```python
from build123d import *

# Parameters (mm, degrees)
EXTRUDE_1_DEPTH      = 3
EXTRUDE_1_DEPTH_BACK = 3
SKETCH_2_W           = 0.5
SKETCH_2_H           = 3
SKETCH_2_H_2         = 1.25
EXTRUDE_2_DEPTH      = 35
SKETCH_3_W           = 6
SKETCH_3_H           = 3
CUT_EXTRUDE_1_DEPTH  = 1.5
CUT_EXTRUDE_2_REACH  = 31.123
SKETCH_4_W           = 0.75
SKETCH_4_H           = 3
SKETCH_2_4_W         = 0.5
SKETCH_2_4_H         = 1.25
EXTRUDE_3_DEPTH      = 4
EXTRUDE_4_REACH      = 40.773
SKETCH_5_W           = 3
SKETCH_5_H           = 3


with BuildPart() as part:
    # Sketch 1 → Extrude 1 (new, two sides: drawn at the far end of the back side and taken through both)
    with BuildSketch(Plane(origin=(0, 0, 0), x_dir=(1, 0, 0), z_dir=(0, 1, 0)).offset(-EXTRUDE_1_DEPTH_BACK)):
        Polygon((-14.75, -19.75), (-14.75, 19.75), (14.75, 19.75), (14.75, -19.75), (15.75, -19.75), (15.75, 23.75), (-15.75, 23.75), (-15.75, -19.75), align=None)
    extrude(amount=EXTRUDE_1_DEPTH + EXTRUDE_1_DEPTH_BACK)

    # Sketch 2 → Extrude 2 (add)
    with BuildSketch(Plane.XY.offset(-19.75)):
        with Locations((-14.5, -1.5)):
            Rectangle(SKETCH_2_W, SKETCH_2_H)
        with Locations((-14.5, 2.375)):
            Rectangle(SKETCH_2_W, SKETCH_2_H_2)
        with Locations((14.5, -1.5)):
            Rectangle(SKETCH_2_W, SKETCH_2_H)
    extrude(amount=EXTRUDE_2_DEPTH)

    # Sketch 3 → Cut-Extrude 1 (cut)
    with BuildSketch(Plane(origin=(0, 0, -23.75), x_dir=(-1, 0, 0), z_dir=(0, 0, -1))):
        with Locations((-9.25, -1.5)):
            Rectangle(SKETCH_3_W, SKETCH_3_H)
        with Locations((9.25, -1.5)):
            Rectangle(SKETCH_3_W, SKETCH_3_H)
    extrude(amount=-CUT_EXTRUDE_1_DEPTH, mode=Mode.SUBTRACT)

    # Sketch 4 → Cut-Extrude 2 (cut, up to next)
    with BuildSketch(Plane(origin=(0, 3, 0), x_dir=(1, 0, 0), z_dir=(0, 1, 0)), mode=Mode.PRIVATE) as cut_extrude_2_sk1:
        with Locations((-15.375, 22.25)):
            Rectangle(SKETCH_4_W, SKETCH_4_H)
    cut_extrude_2_tool1 = extrude(cut_extrude_2_sk1.sketch, amount=-CUT_EXTRUDE_2_REACH, mode=Mode.PRIVATE) & part.part
    add(cut_extrude_2_tool1.solids().sort_by_distance((-15.375, 3, -22.25))[0], mode=Mode.SUBTRACT)

    # Sketch 2_4 → Extrude 3 (add)
    with BuildSketch(Plane.XY.offset(-19.75)):
        with Locations((14.5, 2.375)):
            Rectangle(SKETCH_2_4_W, SKETCH_2_4_H)
    extrude(amount=EXTRUDE_3_DEPTH)

    # Sketch 5 → Extrude 4 (add, up to next)
    with BuildSketch(Plane(origin=(-14.75, 0, 0), x_dir=(0, 0, -1), z_dir=(1, 0, 0)), mode=Mode.PRIVATE) as extrude_4_sk1:
        with Locations((-18.25, -1.5)):
            Rectangle(SKETCH_5_W, SKETCH_5_H)
    extrude_4_tool1 = extrude(extrude_4_sk1.sketch, amount=EXTRUDE_4_REACH, mode=Mode.PRIVATE) - part.part
    add(extrude_4_tool1.solids().sort_by_distance((-14.75, -1.5, 18.25))[0])


solid = part.part
```
Part model, mm, in its own coordinate system. A direction names the side the tool comes from. Coordinates: 2 decimals unless noted, no trailing zeros. Write each loop counter-clockwise with the first axis right and the second up, starting at its lowest first coordinate (ties: lowest second). Pieces come first, ordered by that corner, then holes.
Item 1: Mould opens along X. For faces 1 (the face through (15.75, 0, -2)), 2 (the face through (1, 0, -23.75)), 3 (the face through (-14.25, 2, -2)), 4 (the face through (12.25, -2, -23)) say: released by +X, released by -X, zero draft, split by the parting line, or undercut.
Item 2: Pin check, flat tips, straight feed: pin 1 (1.5 mm diameter, centred on x = -7.5, y = -2, fed in from -Z); pin 2 (1.2 mm diameter, centred on x = 8.5, z = -23, fed in from -Y); pin 3 (1.5 mm diameter, centred on y = 0.5, z = -22.5, fed in from -X). Stop position of each tip, or through.
Item 3: Probe line 1 (X direction, y = 1.8, z = -9.5); line 2 (X direction, y = 1.3, z = -10.5); line 3 (Z direction, x = 3.5, y = -1.65). List the from-to ranges inside material, lowest first.
Item 4: Which spindle directions (+Z, -Z, +X, -X, +Y, -Y) get a long thin tool onto all of the face, cutting with end or side? Do faces 5 (the face through (0, -2, 16.75)), 6 (the face through (14.25, 2, -18)), 7 (the face through (9, -1, -22.25)). Say none if no direction does.
Item 5: Slice it at A-A (z = -2.5). Write the cut outline in (x, y), and give its area (3 significant figures).
Item 6: Slice it at D-D (y = 0.85). Write the cut outline in (x, z), and give its area (3 significant figures).
Item 7: Slice it at B-B (x = 11). Write the cut outline in (y, z).
Item 8: Slice it at C-C (y = -1.9). Write the cut outline in (x, z).
Results found:
1. face 1: released by +X
1. face 2: zero draft
1. face 3: undercut
1. face 4: undercut
2. pin 1: stops at z = -22.25
2. pin 2: stops at y = 0
2. pin 3: stops at x = -15
3. line 1: x = -15.75 to -14.25, 14.75 to 15.75
3. line 2: x = -15.75 to -14.75, 14.75 to 15.75
3. line 3: z = -23.75 to -19.75, 16.75 to 19.75
4. face 5: +Y, -Y
4. face 6: +Z, +Y, -Y
4. face 7: -Z, -Y
5. outline: (-15.75, -3) - (-14.25, -3) - (-14.25, 0) - (-14.75, 0) - (-14.75, 1.75) - (-14.25, 1.75) - (-14.25, 3) - (-15.75, 3) - close; (14.25, -3) - (15.75, -3) - (15.75, 3) - (14.75, 3) - (14.75, 0) - (14.25, 0) - close
5. area: 15.6 mm2
6. outline: (-15.75, -20.75) - (-15, -20.75) - (-15, -23.75) - (15.75, -23.75) - (15.75, 19.75) - (14.75, 19.75) - (14.75, -19.75) - (-14.75, -19.75) - (-14.75, 19.75) - (-15.75, 19.75) - close
6. area: 203 mm2
7. outline: (-3, -22.25) - (0, -22.25) - (0, -23.75) - (3, -23.75) - (3, -19.75) - (-3, -19.75) - close; (-3, 16.75) - (0, 16.75) - (0, 19.75) - (-3, 19.75) - close
8. outline: (-15.75, -20.75) - (-15, -20.75) - (-15, -23.75) - (-12.25, -23.75) - (-12.25, -22.25) - (-6.25, -22.25) - (-6.25, -23.75) - (6.25, -23.75) - (6.25, -22.25) - (12.25, -22.25) - (12.25, -23.75) - (15.75, -23.75) - (15.75, 19.75) - (-15.75, 19.75) - close; hole (-14.75, 15.25) - (-14.25, 15.25) - (-14.25, -19.75) - (14.25, -19.75) - (14.25, 15.25) - (14.75, 15.25) - (14.75, 16.75) - (-14.75, 16.75) - close
